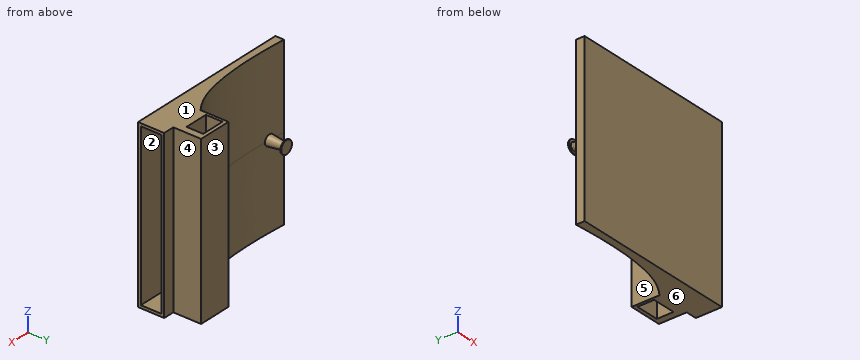
```python
from build123d import *

# Parameters (mm, degrees)
SKETCH1_W           = 49.4
SKETCH1_H           = 140
BOSS_EXTRUDE1_DEPTH = 10
BOSS_EXTRUDE3_DEPTH = 30
SKETCH25_W          = 60
SKETCH25_H          = 9.4
BOSS_EXTRUDE4_DEPTH = 11
SHELL1_T            = -1
SKETCH34_W          = 12
SKETCH34_H          = 60
BOSS_EXTRUDE5_DEPTH = 10
SKETCH38_W          = 8.5
SKETCH38_H          = 6
CUT_EXTRUDE3_DEPTH  = 71.530064661


with BuildPart() as part:
    # Sketch1 → Boss-Extrude1 (new, symmetric)
    with BuildSketch(Plane(origin=(0, 0, 0), x_dir=(1, 0, 0), z_dir=(0, 1, 0))):
        Rectangle(SKETCH1_W, SKETCH1_H)
    extrude(amount=BOSS_EXTRUDE1_DEPTH, both=True)


with BuildPart() as body_2:
    # Sketch5 → Boss-Extrude3 (new, symmetric)
    with BuildSketch(Plane.XY):
        with BuildLine():
            Line((24.7, 0), (24.7, -9.4))
            Line((24.7, -9.4), (-24.7, -9.4))
            Line((-24.7, -9.4), (-24.7, -6.3))
            add(Edge.make_bspline(
                [(19.7, 0), (15.043437724, -3.574706607), (0.818334702, -7.477752328), (-14.226377906, -7.046455079), (-24.7, -6.3)],
                knots=[0, 0, 0, 0, 0.353407129, 1, 1, 1, 1], degree=3))
            Line((19.7, 0), (24.7, 0))
        make_face()
    extrude(amount=BOSS_EXTRUDE3_DEPTH, both=True)


with BuildPart() as part_1:
    add(part.part)

    # Combine1: intersect body 2
    add(body_2.part, mode=Mode.INTERSECT)

    # Sketch8 → Revolve2 (revolve)
    with BuildSketch(Plane.XY, mode=Mode.PRIVATE) as revolve2_sk:
        with BuildLine():
            Line((-20.8, -7.364032413), (-20.06367715, -1.36716404))
            ThreePointArc((-20.06367715, -1.36716404), (-20.111122975, -1.085879422), (-20.30465694, -0.876316193))
            Line((-20.30465694, -0.876316193), (-21.150764231, -0.876316193))
            Line((-21.150764231, -0.876316193), (-21.150764231, -0.535859851))
            Line((-21.150764231, -0.535859851), (-18.8, -0.535859851))
            Line((-18.8, -0.535859851), (-18.8, -0.876316193))
            Line((-18.8, -0.876316193), (-18.8, -7.364032413))
            Line((-18.8, -7.364032413), (-20.8, -7.364032413))
        make_face()
    revolve(revolve2_sk.sketch.rotate(Axis((-18.8, -0.876316193, 0), (0, -1, 0)), 270), axis=Axis((-18.8, -0.876316193, 0), (0, -1, 0)))



with BuildPart() as body_2_2:
    # Sketch25 → Boss-Extrude4 (new body)
    with BuildSketch(Plane(origin=(24.7, 0, 0), x_dir=(0, 0, -1), z_dir=(1, 0, 0))):
        with Locations((0, -4.7)):
            Rectangle(SKETCH25_W, SKETCH25_H)
    extrude(amount=BOSS_EXTRUDE4_DEPTH)

    # Shell1
    shell1_openings = [body_2_2.faces().sort_by_distance(p)[0] for p in [
        (35.7, -4.7, 0),
    ]]
    offset(amount=SHELL1_T, openings=shell1_openings, kind=Kind.INTERSECTION)


with BuildPart() as part_2:
    add(part_1.part)

    add(body_2_2.part)  # Boss-Extrude5 merges body 2 2
    # Sketch34 → Boss-Extrude5 (add)
    with BuildSketch(Plane(origin=(0, 0, 0), x_dir=(1, 0, 0), z_dir=(0, 1, 0))):
        with Locations((25.7, 0)):
            Rectangle(SKETCH34_W, SKETCH34_H)
    extrude(amount=BOSS_EXTRUDE5_DEPTH)

    # Sketch38 → Cut-Extrude3 (cut, through all)
    with BuildSketch(Plane(origin=(0, 0, -30), x_dir=(-1, 0, 0), z_dir=(0, 0, -1))):
        with Locations((-24.948170483, 5.70970961)):
            Rectangle(SKETCH38_W, SKETCH38_H)
    extrude(amount=-CUT_EXTRUDE3_DEPTH, mode=Mode.SUBTRACT)


solid = part_2.part
```
Could you check a few things on this model? Use its own coordinates, in mm. Face numbers are marked on the shaded views. A direction names the side the tool comes from. Round coordinates to 2 decimals unless told otherwise and drop trailing zeros. Loops run counter-clockwise (first coordinate to the right, second up) from the corner with the lowest first, then second, coordinate; pieces in that order, holes last. Notation, with made-up numbers: (-16, 56.25) - (7, 56.25) arc R29 cw to (7, 77.25) - close; hole circle Ø7 at (85, -31.5). An arc over 180 degrees is marked (long way). Answer as CSV lines item,"result".
1. Please list where these lines run through material, in increasing order: line 1 along X through (y, z) = (5.25, 2); line 2 along Y through (x, z) = (24, -16); line 3 along Y through (x, z) = (17.5, -27). Write a range as [from, to].
Filled in:
line 1,"x = [19.7, 20.7], [29.2, 31.7]"
line 2,"y = [-9.4, 2.71], [8.71, 10]"
line 3,"y = [-9.4, -1.52]"
2. We'd pull the mould along Z, two halves only. Please class the marked faces 1, 2 and 3: +Z half, -Z half, draft (parallel to the pull), parting line (faces both ways), or undercut.
Filled in:
face 1,"+Z half"
face 2,"undercut"
face 3,"draft"
3. I want a section at B-B on x = 24. List the corners of the cut face in (y, z) for me.
Filled in:
outline,"(-9.4, -30) - (2.71, -30) - (2.71, 30) - (-9.4, 30) - close; (8.71, -30) - (10, -30) - (10, 30) - (8.71, 30) - close"
4. I want a section at A-A on y = 4.25. List the corners of the cut face in (x, z) for me, then the cut area to 3 significant figures.
Filled in:
outline,"(19.7, -30) - (20.7, -30) - (20.7, 30) - (19.7, 30) - close; (29.2, -30) - (31.7, -30) - (31.7, 30) - (29.2, 30) - close"
area,"210 mm^2"
5. On a 3-axis mill with a long thin cutter (end or side, diameter ignored), from which of +Z, -Z, +X, -X, +Y, -Y can I reach the whole of each face in a straight line? I mean the marked faces 4, 5 and 6. Say none if no direction works.
Filled in:
face 4,"+Z, -Z, +X, +Y"
face 5,"+Z, -Z, -X, +Y"
face 6,"-Z, +X, -X, +Y, -Y"
6. For pin 1 Ø1.5 at (y, z) = (2, 23.5) entering from -X; pin 2 Ø3 at (y, z) = (5, 3) entering from +X; pin 3 Ø4.5 at (x, z) = (34.5, -12.5) entering from +Y, each with a flat end and sliding along its axis, tell me the tip position at first contact or that it passes through.
Filled in:
pin 1,"stops at x = 19.7"
pin 2,"stops at x = 31.7"
pin 3,"stops at y = 0"
